Can you work these out from the model? Positions are in its coordinate system, mm. Give positions to 0.01 mm unless a question says otherwise; leave off trailing zeros. Loops run counter-clockwise (first coordinate to the right, second up) from the corner with the lowest first, then second, coordinate; pieces in that order, holes last. Notation, with made-up numbers: (75, 61.5) -> (100, 61.5) arc R16 cw to (100, 90.5) -> close; hole circle Ø6 at (30.25, 45.5). An arc over 180 degrees is marked (long way). One line per question, with ' | ' between items.
from build123d import *

# Parameters (mm, degrees)
F0_W     = 444.5
F0_H     = 127
F1_DEPTH = 3.175
F2_R     = 2.5527
F2_R_2   = 2.4892
F3_DEPTH = 25.4
F5_DEPTH = 444.501


# Not quite as in the source:
# - a feature names something its author has since deleted; it is built from what else it names


with BuildPart() as f1:
    # F0 (on Top) → F1 (new body)
    with BuildSketch(Plane.XY):
        with Locations((222.25, -63.5)):
            Rectangle(F0_W, F0_H)
    extrude(amount=F1_DEPTH)

    # F2 (on face) → F3 (cut)
    with BuildSketch(Plane.XY.offset(3.175)):
        with Locations((12.7, -104.1527)):
            Circle(F2_R)
        with Locations((12.7, -91.4527)):
            Circle(F2_R)
        with Locations((12.7, -78.7527)):
            Circle(F2_R)
        with Locations((12.7, -66.0527)):
            Circle(F2_R)
        with Locations((12.7, -53.3527)):
            Circle(F2_R)
        with Locations((431.8, -101.6)):
            Circle(F2_R_2)
        with Locations((431.8, -88.9)):
            Circle(F2_R_2)
        with Locations((431.8, -76.2)):
            Circle(F2_R_2)
        with Locations((431.8, -63.5)):
            Circle(F2_R_2)
        with Locations((431.8, -50.8)):
            Circle(F2_R_2)
        with Locations((12.7, -40.6527)):
            Circle(F2_R)
        with Locations((431.8, -38.1)):
            Circle(F2_R_2)
    extrude(amount=-F3_DEPTH, mode=Mode.SUBTRACT)

    # F4 (on face) → F5 (cut, through all)
    with BuildSketch(Plane.YZ.offset(444.5)):
        Polygon((-95.25, 0), (-120.65, 3.175), (-127, 3.175), (-127, 0), align=None)
    extrude(amount=-F5_DEPTH, mode=Mode.SUBTRACT)


solid = f1.part
Q1. If we section it at A-A (z = 2.25): State how many separate pieces and enclosed holes the cut face has, plus the area to 3 significant figures.
Entries:
separate pieces: 1 | enclosed holes: 12 | area: 50,100 mm²
Q2. If I drill on probe 1 along Y at (x, z) = (12.7, 1.2); probe 2 along X at (y, z) = (-76.5, 2.9); probe 3 along Z at (x, y) = (386, -107.5) (3 decimals), over which ranges is the centre line in solid material (lowest first)? Write a range as from..to.
Entries:
probe 1: -101.6..-94.01, -88.9..-81.31, -76.2..-68.61, -63.5..-55.91, -50.8..-43.21, -38.1..0 | probe 2: 0..11.5, 13.9..429.33, 434.27..444.5 | probe 3: 1.531..3.175
Q3. For pin 1 Ø6.5 at (x, y) = (431.8, -50.8) entering from -Z, with a flat end and sliding along its axis, tell me the tip position at first contact or that it passes through.
Entries:
pin 1: z = 0
Q4. If we section it at B-B (x = 281.5): Write out the boundary of the cut face in (y, z) (3 decimals).
Entries:
outline: (-120.65, 3.175) -> (-95.25, 0) -> (0, 0) -> (0, 3.175) -> close
